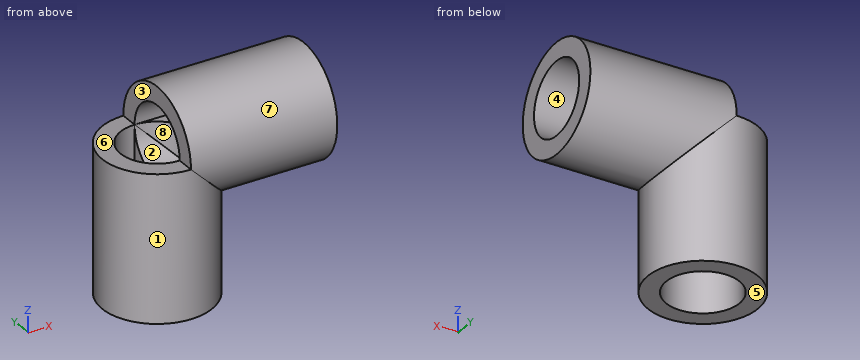
Autodesk Inventor part; units mm, degrees
ref_plane "YZ Plane" through (0, 0, 0) normal (1, 0, 0) x (0, 1, 0)
ref_plane "XZ Plane" through (0, 0, 0) normal (0, 1, 0) x (-1, 0, 0)
ref_plane "XY Plane" through (0, 0, 0) normal (0, 0, 1) x (1, 0, 0)
sketch "Sketch1" plane through (0, 0, 0) normal (0, 0, 1) x (1, 0, 0)
  circle A0 centre (0, 0) radius 5
  circle A1 centre (0, 0) radius 7.5
  dimension "d0" = 10
  dimension "d1" = 15
extrude "Extrusion1" add sketch "Sketch1" along normal blind 20
sketch "Sketch2" plane through (0, 0, 0) normal (1, 0, 0) x (0, 1, 0)
  line L0 (7.5, 20) -> (-7.5, 20)
  circle A0 centre (0, 20) radius 5
  circle A1 centre (0, 20) radius 7.5
  point P0 (0, 0)
  dimension "d4" = 10
  dimension "d5" = 15
extrude "Extrusion2" add sketch "Sketch2" along normal blind 20 contours A1 L0 A0 | L0 A0 A1
properties part number "ccccccc"
The model under review builds one solid part; all positions refer to its coordinate system, in mm. Face numbers are marked on the shaded views. A direction names the side the tool comes from. Round coordinates to 2 decimals unless told otherwise and drop trailing zeros. Loops run counter-clockwise (first coordinate to the right, second up) from the corner with the lowest first, then second, coordinate; pieces in that order, holes last.
1) Tool access review of the marked faces 1, 2, 3, 4 and 5: name each direction out of +Z, -Z, +X, -X, +Y, -Y from which nothing blocks a thin tool from reaching the whole face with its end or side.
Values follow:
face 1: -Z
face 2: none
face 3: +Z, -X, +Y, -Y
face 4: +X
face 5: -Z, +X, -X, +Y, -Y
2) Consider section A-A on y = 0. State the section outline as (x, z) points.
Values follow:
outline: (-7.5, 0) - (-5, 0) - (-5, 20) - (-7.5, 20) - close; (0, 12.5) - (5, 12.5) - (5, 0) - (7.5, 0) - (7.5, 12.5) - (20, 12.5) - (20, 15) - (7.5, 15) - (7.5, 20) - (5, 20) - (5, 15) - (0, 15) - close; (0, 25) - (20, 25) - (20, 27.5) - (0, 27.5) - close
3) Consider section B-B on z = 13.25. State the section outline as (x, y) points.
Values follow:
outline: (6.75, -3.27) - (20, -3.27) - (20, 3.27) - (6.75, 3.27) arc R7.5 ccw (long way) to start; hole (0, -3.27) - (0, 3.27) - (3.78, 3.27) arc R5 ccw (long way) to (3.78, -3.27) - close
4) Consider section D-D on z = 24.5. State the section outline as (x, y) points, then the cut area to 3 significant figures.
Values follow:
outline: (0, -6) - (20, -6) - (20, -2.18) - (0, -2.18) - close; (0, 2.18) - (20, 2.18) - (20, 6) - (0, 6) - close
area: 153 mm2
5) The part is to be moulded in two halves that separate along Y. For the marked faces 6, 7 and 8, say which applies: pulls with the +Y half, pulls with the -Y half, needs draft (parallel to the pull), parting line crosses it, or undercut.
Values follow:
face 6: needs draft
face 7: parting line crosses it
face 8: undercut
6) Wall thickness on line 1 along Z through (x, y) = (7.75, 0); line 2 along X through (y, z) = (0, 13.5); line 3 along Y through (x, z) = (1.25, 13.5): over which ranges is each line inside the solid? List them lowest first.
Values follow:
line 1: z = 12.5 to 15, 25 to 27.5
line 2: x = -7.5 to -5, 0 to 20
line 3: y = -7.4 to -4.84, -3.74 to 3.74, 4.84 to 7.4
7) Consider section C-C on x = -1.75. State the section outline as (y, z) points.
Values follow:
outline: (-7.29, 0) - (-4.68, 0) - (-4.68, 20) - (-7.29, 20) - close; (4.68, 0) - (7.29, 0) - (7.29, 20) - (4.68, 20) - close
8) Clearance check with flat-ended pins moving along their axes: P1, Ø4, axis at y = -5.5, z = 8, coming from the +X side; P2, Ø3, axis at y = 2, z = 16.5, coming from the -X side; P3, Ø6, axis at y = -2.5, z = 25, coming from the -X side. State where each tip first meets the part, or that it passes through.
Values follow:
P1: stops at x = 6.63
P2: stops at x = -7.48
P3: stops at x = 0
